Autodesk Inventor part; units mm, degrees
ref_plane "YZ Plane" through (0, 0, 0) normal (1, 0, 0) x (0, 1, 0)
ref_plane "XZ Plane" through (0, 0, 0) normal (0, 1, 0) x (-1, 0, 0)
ref_plane "XY Plane" through (0, 0, 0) normal (0, 0, 1) x (1, 0, 0)
sketch "Sketch1" plane through (0, 0, 0) normal (0, 1, 0) x (-1, 0, 0)
  circle A0 centre (0, 0) radius 4
  dimension "d0" = 8
extrude "Extrusion1" add sketch "Sketch1" along normal blind 6
sketch "Sketch2" plane through (0, 6, 0) normal (0, 1, 0) x (1, 0, 0)
  circle A0 centre (0, 0) radius 4
  circle A1 centre (0, 0) radius 3
  dimension "d3" = 6
extrude "Extrusion2" cut sketch "Sketch2" against normal up to next contours A1
chamfer "Chamfer1" distance 0.5 angle 45 1 edges at (-3, 6, 0)
properties part number "E3DBowdenInsert" material "Brass, Soft Yellow"
For this review, take the finished solid that the model builds, in its own axes (mm). Round coordinates to 2 decimals unless told otherwise and drop trailing zeros. Write each loop counter-clockwise with the first axis right and the second up, starting at its lowest first coordinate (ties: lowest second). Pieces come first, ordered by that corner, then holes. Notation, with made-up numbers: (-39.75, -16) - (-8.75, -16) arc R26 ccw to (-8.75, -2) - close; hole circle Ø10 at (76, 77.25). An arc over 180 degrees is marked (long way). Write item = value, one per line. Start each with the question number.
1. For pin 1 Ø1.5 at (y, z) = (5, 2) entering from +X; pin 2 Ø1 at (x, y) = (-2, 5) entering from -Z, all flat-tipped, find the tip position at first contact; note any pin that passes through.
2. Consider section A-A on x = 0. State the section outline as (y, z) points.
3. Consider section B-B on z = 0. State the section outline as (x, y) points, plus the area to 4 significant figures.
4. Consider section C-C on y = 3.55. State the section outline as (x, z) points, plus the area to 3 significant figures.
5. Draft analysis for pull direction Z (two halves, no side actions). For faces 1 (the face through (-3, 3, 0)), 2 (the face through (0.867, 2.958, 3.905)), 3 (the face through (-1, 0, 3)), state which applies: released by +Z, released by -Z, zero draft, split by the parting line, or undercut.
6. Wall thickness on L1, parallel to Z at x = 0, y = 3.5; L2, parallel to Z at x = 1, y = 0.8; L3, parallel to X at y = 4.8, z = 2.5: over which ranges is each line inside the solid? List them lowest first.
Evaluation:
q1.pin_1 = 3.8
q1.pin_2 = -3.71
q2.outline = (0, -4) - (6, -4) - (6, -3.5) - (5.5, -3) - (0, -3) - close; (0, 3) - (5.5, 3) - (6, 3.5) - (6, 4) - (0, 4) - close
q3.outline = (-4, 0) - (-3, 0) - (-3, 5.5) - (-3.5, 6) - (-4, 6) - close; (3, 0) - (4, 0) - (4, 6) - (3.5, 6) - (3, 5.5) - close
q3.area = 11.75 mm2
q4.outline = circle Ø8 at (0, 0); hole circle Ø6 at (0, 0)
q4.area = 22.0 mm2
q5.face_1 = undercut
q5.face_2 = split by the parting line
q5.face_3 = zero draft
q6.L1 = -4 to -3, 3 to 4
q6.L2 = -3.87 to -2.83, 2.83 to 3.87
q6.L3 = -3.12 to -1.66, 1.66 to 3.12
